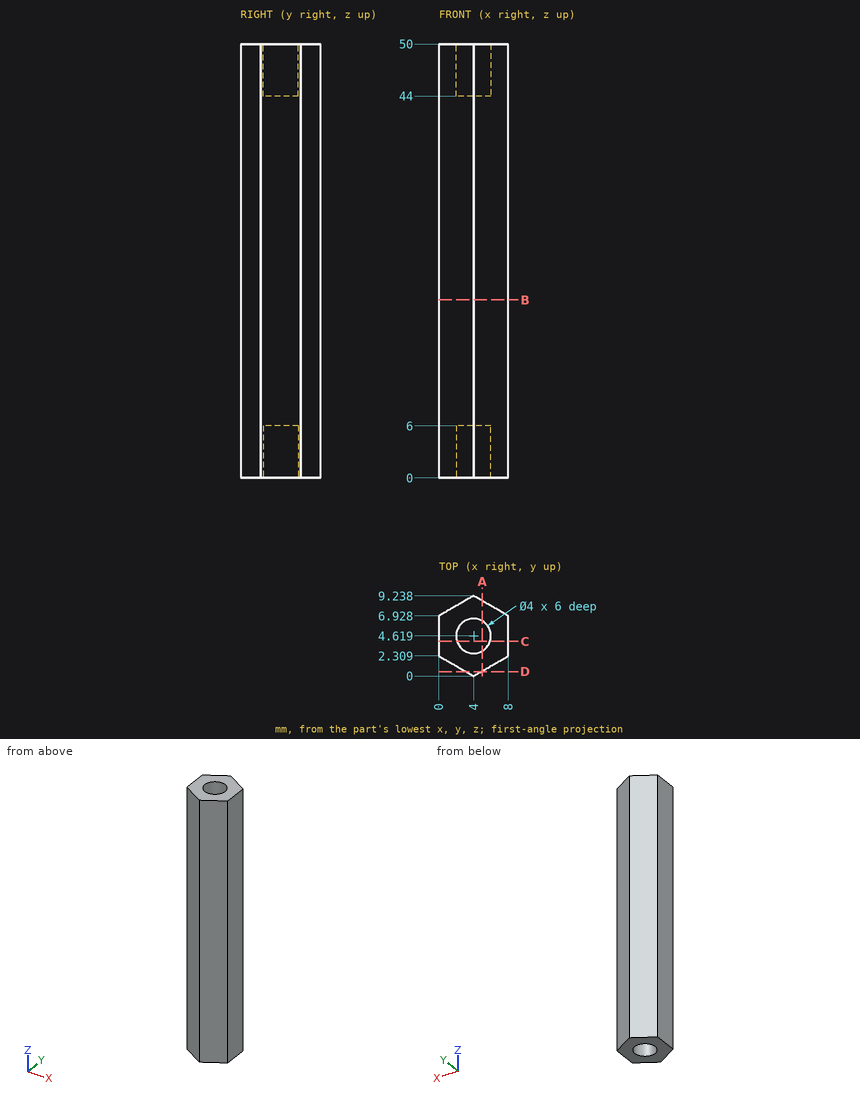
Verification items for this drawing (mm, ordinates from the low corner). Give positions to 0.01 mm unless a question says otherwise; leave off trailing zeros. Write each loop counter-clockwise with the first axis right and the second up, starting at its lowest first coordinate (ties: lowest second). Pieces come first, ordered by that corner, then holes. Notation, with made-up numbers: (71, -30) -> (94, -30) arc R23 cw to (94, -1) -> close; hole circle Ø1 at (60, 81.5). An arc over 180 degrees is marked (long way). Write item = value, one per line.
Item 1: Sectioned sample at D-D on y = 0.5. Record the boundary of the cut face in (x, z).
Output:
outline = (3.13, 0) -> (4.87, 0) -> (4.87, 50) -> (3.13, 50) -> close
Item 2: Sectioned sample at C-C on y = 4. Record the boundary of the cut face in (x, z), and give its area (3 significant figures).
Output:
outline = (0, 0) -> (2.1, 0) -> (2.1, 6) -> (5.9, 6) -> (5.9, 0) -> (8, 0) -> (8, 50) -> (5.9, 50) -> (5.9, 44) -> (2.1, 44) -> (2.1, 50) -> (0, 50) -> close
area = 354 mm^2
Item 3: Scan lines: probe 1 along Y at (x, z) = (4, 46.9); probe 2 along Z at (x, y) = (4.75, 5); probe 3 along X at (y, z) = (5.25, 4.5). Record each from-to range of solid material in increasing order. Write a range as from..to.
Output:
probe_1 = 0..2.62, 6.62..9.24
probe_2 = 6..44
probe_3 = 0..2.1, 5.9..8
Item 4: Gauge pin test, flat ends, axial feed: pin 1 (3 mm diameter, centred on x = 4, y = 4.62, fed in from +Z); pin 2 (1 mm diameter, centred on y = 7.5, z = 32, fed in from +X) (1 decimal). Record the tip position at first contact, or that the pin passes through.
Output:
pin_1 = 44
pin_2 = 7.9
Item 5: Sectioned sample at A-A on x = 5. Record the boundary of the cut face in (y, z).
Output:
outline = (0.58, 0) -> (2.89, 0) -> (2.89, 6) -> (6.35, 6) -> (6.35, 0) -> (8.66, 0) -> (8.66, 50) -> (6.35, 50) -> (6.35, 44) -> (2.89, 44) -> (2.89, 50) -> (0.58, 50) -> close
Item 6: Sectioned sample at B-B on z = 20.5. Record the boundary of the cut face in (x, y), and give its area (3 significant figures).
Output:
outline = (0, 2.31) -> (4, 0) -> (8, 2.31) -> (8, 6.93) -> (4, 9.24) -> (0, 6.93) -> close
area = 55.4 mm^2
